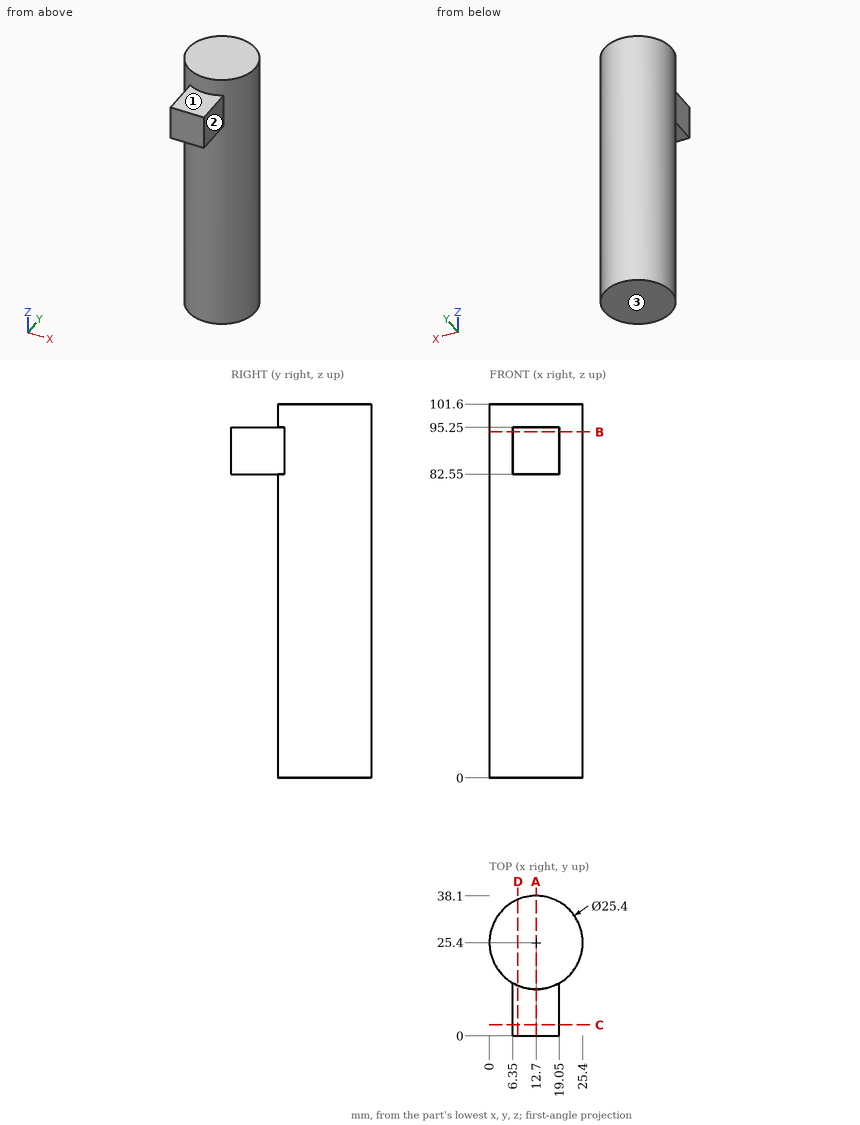
Source: three-view drawing plus pictorial views. Frame: mm from the lowest corner of the part. Coordinates: 2 decimals unless noted, no trailing zeros. Order: outer loops, then holes, each group sorted by start corner. A loop starts at its lowest first (then second) coordinate and runs counter-clockwise, first axis right, second up.
1) Ray query, probe 1 along Z at (x, y) = (18.75, 2); probe 2 along Y at (x, z) = (19, 75); probe 3 along X at (y, z) = (18, 18). Return the intervals inside material, ascending.
Result sheet:
probe 1: z = 82.55 to 95.25
probe 2: y = 14.37 to 36.43
probe 3: x = 2.38 to 23.02
2) Section C-C (y = 3). Return loops of the section in (x, z), then the cut area to 3 significant figures.
Result sheet:
outline: (6.35, 82.55) - (19.05, 82.55) - (19.05, 95.25) - (6.35, 95.25) - close
area: 161 mm2
3) Section D-D (x = 7.75). Return loops of the section in (y, z).
Result sheet:
outline: (0, 82.55) - (13.7, 82.55) - (13.7, 0) - (37.1, 0) - (37.1, 101.6) - (13.7, 101.6) - (13.7, 95.25) - (0, 95.25) - close
4) Section B-B (z = 94). Return loops of the section in (x, y), then the cut area to 3 significant figures.
Result sheet:
outline: (6.35, 0) - (19.05, 0) - (19.05, 14.4) arc R12.7 ccw (long way) to (6.35, 14.4) - close
area: 675 mm2
5) Section A-A (x = 12.7). Return loops of the section in (y, z), then the cut area to 3 significant figures.
Result sheet:
outline: (0, 82.55) - (12.7, 82.55) - (12.7, 0) - (38.1, 0) - (38.1, 101.6) - (12.7, 101.6) - (12.7, 95.25) - (0, 95.25) - close
area: 2,740 mm2
6) Draft query along Z for the marked faces 1, 2 and 3. Return one class per face: released by +Z, released by -Z, zero draft, split by the parting line, or undercut.
Result sheet:
face 1: released by +Z
face 2: zero draft
face 3: released by -Z
7) First-contact query: P1, Ø1, axis at y = 29.5, z = 20.5, coming from the +X side; P2, Ø6, axis at y = 31, z = 44, coming from the -X side; P3, Ø12, axis at x = 5, z = 25, coming from the +Y side. Flat tips, straight axial feed; report the tip coordinate or a pass-through.
Result sheet:
P1: stops at x = 24.88
P2: stops at x = 0.27
P3: stops at y = 37.99
